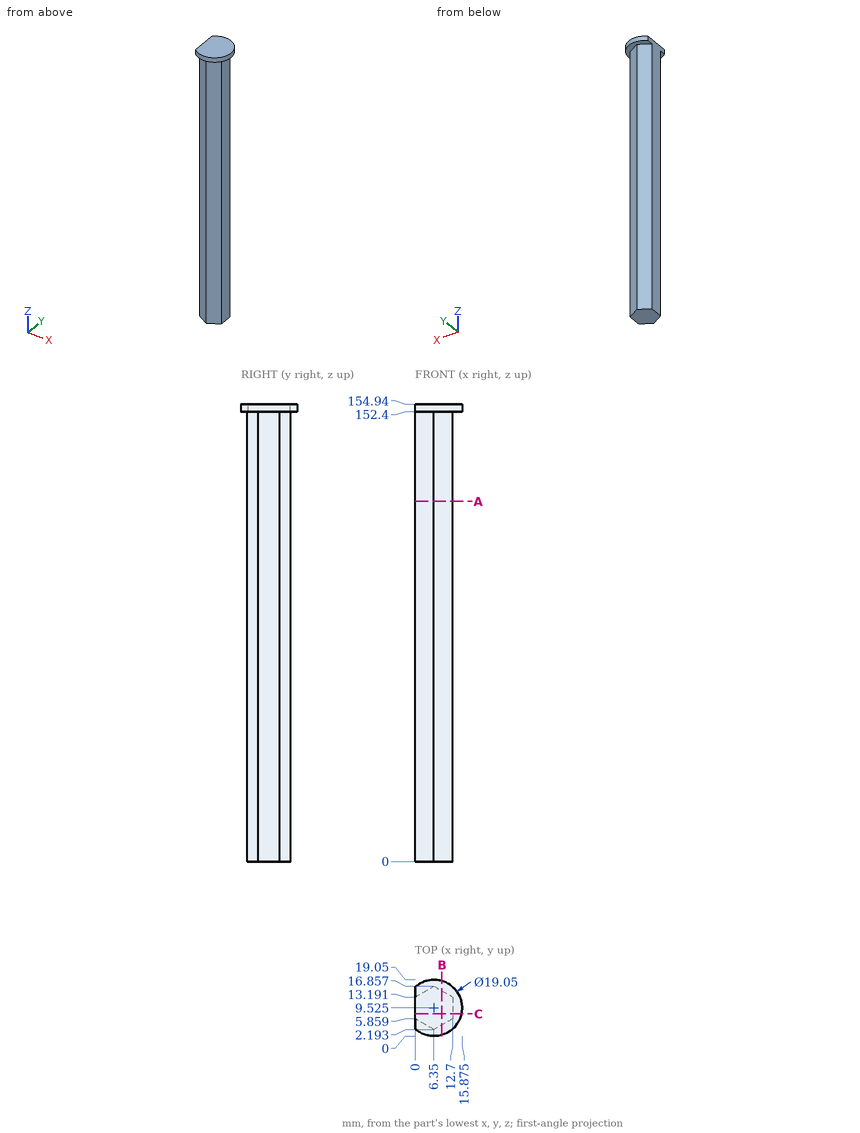
For this review, use the dimensioned drawing (mm, ordinates from the lowest corner) and the shaded views. Coordinates: 2 decimals unless noted, no trailing zeros. Order: outer loops, then holes, each group sorted by start corner. A loop starts at its lowest first (then second) coordinate and runs counter-clockwise, first axis right, second up. Notation, with made-up numbers: (-34, 62) - (-17, 62) arc R17 cw to (-17, 79) - close; hole circle Ø10 at (-4.75, 13). An arc over 180 degrees is marked (long way). Answer as a JSON object with one key per item and string values. Group by question number.
1. We need section C-C on y = 7.5. State the section outline as (x, z) points.
2. We need section A-A on z = 122. State the section outline as (x, y) points, then the cut area to 3 significant figures.
3. Clearance check with flat-ended pins moving along their axes: P1, Ø6, axis at y = 11.5, z = 65, coming from the +X side; P2, Ø8, axis at x = 13.5, z = 40, coming from the +Y side; P3, Ø6, axis at x = 3.5, z = 108.5, coming from the -Y side. State where each tip first meets the part, or that it passes through.
4. For probe 1 along X at (y, z) = (8.5, 31.5); probe 2 along Z at (x, y) = (3, 18.25); probe 3 along X at (y, z) = (15, 123) (1 decimal), list the stretches that pass through material, from the lowest coordinate up.
5. We need section B-B on x = 9. State the section outline as (y, z) points.
Final values:
{
 "1": {"outline": "(0, 0) - (12.7, 0) - (12.7, 152.4) - (15.66, 152.4) - (15.66, 154.94) - (0, 154.94) - close"},
 "2": {"outline": "(0, 5.86) - (6.35, 2.19) - (12.7, 5.86) - (12.7, 13.19) - (6.35, 16.86) - (0, 13.19) - close", "area": "140 mm²"},
 "3": {"P1": "x = 12.7", "P2": "y = 15.04", "P3": "y = 2.19"},
 "4": {"probe 1": "0 to 12.7", "probe 2": "152.4 to 154.94", "probe 3": "3.1 to 9.6"},
 "5": {"outline": "(0.38, 152.4) - (3.72, 152.4) - (3.72, 0) - (15.33, 0) - (15.33, 152.4) - (18.67, 152.4) - (18.67, 154.94) - (0.38, 154.94) - close"}
}
